Work out the finished part from the listing and answer in its coordinate system (mm). Face numbers are marked on the shaded views. A direction names the side the tool comes from. Round coordinates to 2 decimals unless told otherwise and drop trailing zeros. Write each loop counter-clockwise with the first axis right and the second up, starting at its lowest first coordinate (ties: lowest second). Pieces come first, ordered by that corner, then holes.
from build123d import *

# Parameters (mm, degrees)
SKETCH_1_R          = 10
EXTRUDE_1_DEPTH     = 16.4
SKETCH_2_R          = 8.85
CUT_EXTRUDE_1_DEPTH = 0.7
SKETCH_3_R          = 1.325
EXTRUDE_2_DEPTH     = 5
CHAMFER_1_SIZE      = 0.8
SKETCH_4_R          = 8.05
CUT_EXTRUDE_2_DEPTH = 1.5
SKETCH_5_R          = 0.6
CUT_EXTRUDE_3_DEPTH = 3
FILLET_1_R          = 0.8


with BuildPart() as part:
    # Эскиз1 → Бобышка-Вытянуть1 (new body)
    with BuildSketch(Plane.XY):
        Circle(SKETCH_1_R)
    extrude(amount=EXTRUDE_1_DEPTH)

    # Эскиз2 → Вырез-Вытянуть1 (cut)
    with BuildSketch(Plane.XY.offset(16.4)):
        Circle(SKETCH_2_R)
    extrude(amount=-CUT_EXTRUDE_1_DEPTH, mode=Mode.SUBTRACT)

    # Эскиз3 → Бобышка-Вытянуть2 (add)
    with BuildSketch(Plane.XY.offset(15.7)):
        with Locations((-4.775, 4.775)):
            Circle(SKETCH_3_R)
        with Locations((-4.775, -4.775)):
            Circle(SKETCH_3_R)
        with Locations((4.775, 4.775)):
            Circle(SKETCH_3_R)
    extrude(amount=EXTRUDE_2_DEPTH)

    # Фаска1
    chamfer_1_edges = [part.edges().sort_by_distance(p)[0] for p in [
        (-6.1, 4.775, 20.7),
        (-6.1, -4.775, 20.7),
        (3.45, 4.775, 20.7),
    ]]
    chamfer(chamfer_1_edges, length=CHAMFER_1_SIZE)

    # Эскиз4 → Вырез-Вытянуть2 (cut)
    with BuildSketch(Plane(origin=(0, 0, 0), x_dir=(-1, 0, 0), z_dir=(0, 0, -1))):
        Circle(SKETCH_4_R)
    extrude(amount=-CUT_EXTRUDE_2_DEPTH, mode=Mode.SUBTRACT)

    # Эскиз5 → Вырез-Вытянуть3 (cut)
    with BuildSketch(Plane(origin=(0, 0, 1.5), x_dir=(-1, 0, 0), z_dir=(0, 0, -1))):
        Circle(SKETCH_5_R)
    extrude(amount=-CUT_EXTRUDE_3_DEPTH, mode=Mode.SUBTRACT)

    # Скругление1
    fillet_1_edges = [part.edges().sort_by_distance(p)[0] for p in [
        (-10, 0, 0),
        (-10, 0, 16.4),
    ]]
    fillet(fillet_1_edges, radius=FILLET_1_R)


solid = part.part
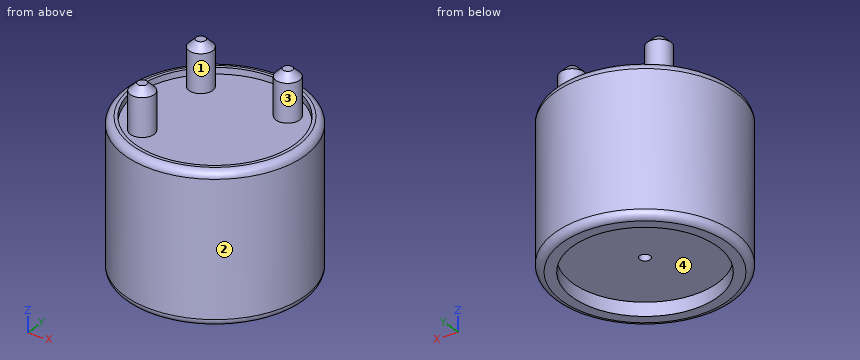
Q1. Find section A-A (x = 0). Determine the outline of the cut face in (y, z), plus the area to 3 significant figures.
Q2. Find section C-C (z = 15.25). Determine the outline of the cut face in (x, y).
Q3. The mould has two halves that part along Y. Classify the marked faces 1 and 2: +Y half, -Y half, draft (parallel to the pull), parting line (faces both ways), or undercut.
Q4. A tool of negligible diameter and unlimited length cuts with its end or side. For the marked faces 3 and 4, from which of +Z, -Z, +X, -X, +Y, -Y can it reach the whole face along a straight path? Write none if from no direction.
Q5. Given pin 1 (3 mm diameter, centred on y = -5.5, z = 4.5, fed in from +X); pin 2 (5 mm diameter, centred on x = -1.5, y = -2.5, fed in from -Z); pin 3 (1.5 mm diameter, centred on x = -0.5, y = 0.5, fed in from +Z), each flat-ended and moving along its own axis, determine where each tip first touches the part or whether it passes through.
Q6. Find the intervals of material crossed by L1, parallel to Y at x = 0, z = 0.8; L2, parallel to Y at x = 0, z = 2.3; L3, parallel to Z at x = -5, y = 0, in increasing order.
Report:
1. outline: (-10, 0.8) arc R0.8 ccw to (-9.2, 0) - (-8.05, 0) - (-8.05, 1.5) - (-0.6, 1.5) - (-0.6, 4.5) - (0.6, 4.5) - (0.6, 1.5) - (8.05, 1.5) - (8.05, 0) - (9.2, 0) arc R0.8 ccw to (10, 0.8) - (10, 15.6) arc R0.8 ccw to (9.2, 16.4) - (8.85, 16.4) - (8.85, 15.7) - (-8.85, 15.7) - (-8.85, 16.4) - (-9.2, 16.4) arc R0.8 ccw to (-10, 15.6) - close
1. area: 287 mm2
2. outline: circle Ø20 at (0, 0)
3. face 1: undercut
3. face 2: parting line
4. face 3: +Z
4. face 4: -Z
5. pin 1: stops at x = 9.17
5. pin 2: stops at z = 1.5
5. pin 3: stops at z = 15.7
6. L1: y = -10 to -8.05, 8.05 to 10
6. L2: y = -10 to -0.6, 0.6 to 10
6. L3: z = 1.5 to 15.7
